Part model, mm, in its own coordinate system. Face numbers are marked on the shaded views. Coordinates: 2 decimals unless noted, no trailing zeros. Write each loop counter-clockwise with the first axis right and the second up, starting at its lowest first coordinate (ties: lowest second). Pieces come first, ordered by that corner, then holes. Notation, with made-up numbers: M 80.5,-28 L 132.5,-28 A35 cw 132.5,11 Z; hole C -34,58.25 d10. An arc over 180 degrees is marked long. Use a Markdown table: item, result. Add a question column.
Q1. Wall check: L1, parallel to Z at x = 20, y = -4.25; L2, parallel to Z at x = 18.5, y = -3; L3, parallel to Y at x = 96.5, z = -6. Give the ranges that are in metal, low to high. Write a range as from..to.
Q2. Slice it at A-A on x = 56.5. Write the cut outline in (y, z).
Q3. Mould opens along Z. For the marked faces 1, 2 and 3 say: released by +Z, released by -Z, zero draft, split by the parting line, or undercut.
Q4. Pin check, flat tips, straight feed: pin 1 Ø4 at (x, z) = (66, 4.5) entering from -Y; pin 2 Ø0.9 at (y, z) = (1, 5.5) entering from +X; pin 3 Ø3 at (x, y) = (61, -6) entering from +Z. Stop position of each tip, or through.
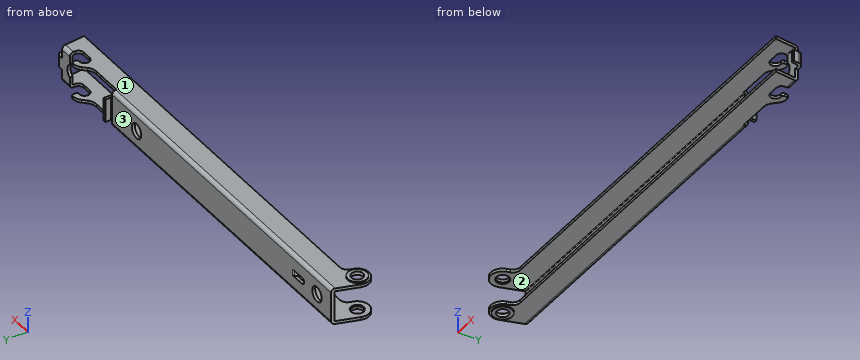
from build123d import *
from OCP.BRepFilletAPI import BRepFilletAPI_MakeFillet

# Parameters (mm, degrees)
BOSS_EXTRUDE1_DEPTH = 6.35
SKETCH2_R           = 3.2766
BOSS_EXTRUDE2_DEPTH = 0.381
FILLET1_R1          = 1.27
FILLET1_R2          = 2.54
SHELL1_T            = -1.016
BOSS_EXTRUDE3_DEPTH = 6.35
FILLET2_R           = 1.27
SHELL2_START        = 118.3386
SHELL2_DEPTH        = 27.813
SHELL2_START_2      = 129.293990182
SHELL2_2_DEPTH      = 7.764409818
FILLET3_R           = 0.635
SKETCH4_R           = 2.032
CUT_EXTRUDE1_DEPTH  = 148.431229717
EXTRUDE_THIN1_DEPTH = 2.0066
CUT_EXTRUDE2_DEPTH  = 150.225017324
EXTRUDE_THIN2_DEPTH = 4.0005
SKETCH8_R           = 2.54
CUT_EXTRUDE3_DEPTH  = 150.217877052
EXTRUDE_THIN3_DEPTH = 1.0795
FILLET4_R           = 0.635
FILLET6_RADIUS      = 1.0795
FILLET6_LENGTH      = 1.016


# Read off the part's stored shape, not the designer's step: Shell2
with BuildPart() as part:
    # Sketch1 → Boss-Extrude1 (new, symmetric)
    with BuildSketch(Plane.XY):
        with BuildLine():
            Line((0, 0), (118.3386, 0))
            Line((118.3386, 0), (118.3386, -8.128))
            Line((118.3386, -8.128), (5.974494608, -8.128))
            Line((5.974494608, -8.128), (5.047186378, -11.093494156))
            ThreePointArc((5.047186378, -11.093494156), (-0.044494156, -13.759386378), (-2.710386378, -8.667705844))
            Line((-2.710386378, -8.667705844), (0, 0))
        make_face()
    extrude(amount=BOSS_EXTRUDE1_DEPTH, both=True)

    # Sketch2 → Boss-Extrude2 (add)
    with BuildSketch(Plane.XY.offset(6.35)):
        with Locations(Location((1.1684, -9.8806, 0), (0, 0, 180))):
            Circle(SKETCH2_R)
    boss_extrude2 = extrude(amount=BOSS_EXTRUDE2_DEPTH)

    # Mirror1: Boss-Extrude2 across plane
    add(boss_extrude2.mirror(Plane.XY))

    # Fillet1: one fillet with a radius per group of edges: ONE call of the kernel's fillet builder (fillet() takes one radius for all edges)
    fillet1_edges_1 = [part.edges().sort_by_distance(p)[0] for p in [
        (59.1693, 0, 6.35),
        (59.1693, 0, -6.35),
    ]]
    fillet1_edges_2 = [part.edges().sort_by_distance(p)[0] for p in [
        (5.974494608, -8.128, 0),
    ]]
    fillet1 = BRepFilletAPI_MakeFillet(part.part.solid().wrapped)
    for e in fillet1_edges_1:
        fillet1.Add(FILLET1_R1, e.wrapped)
    for e in fillet1_edges_2:
        fillet1.Add(FILLET1_R2, e.wrapped)
    add(Compound.cast(fillet1.Shape()), mode=Mode.REPLACE)

    # Shell1
    shell1_openings = [part.faces().sort_by_distance(p)[0] for p in [
        (118.3386, -4.089523172, 0),
        (63.090062087, -8.128, 0),
        (5.232234532, -10.501717654, 0),
        (-0.044494156, -13.759386378, 0),
        (-1.363208192, -4.359484576, 0),
        (6.337175389, -8.621408996, 0),
    ]]
    offset(amount=SHELL1_T, openings=shell1_openings, kind=Kind.INTERSECTION)

    # Sketch3 → Boss-Extrude3 (add, symmetric)
    with BuildSketch(Plane.XY):
        with BuildLine():
            Line((118.3386, -8.128), (146.1516, -8.128))
            Line((146.1516, -8.128), (145.2626, 0.0762))
            Line((145.2626, 0.0762), (141.1224, 0.0762))
            Line((141.1224, 0.0762), (141.1224, -1.8034))
            ThreePointArc((141.1224, -1.8034), (140.594196369, -3.078596369), (139.319, -3.6068))
            Line((139.319, -3.6068), (136.0678, -3.6068))
            ThreePointArc((136.0678, -3.6068), (134.2644, -1.8034), (136.0678, 0))
            Line((136.0678, 0), (137.0584, 0))
            Line((137.0584, 0), (137.0584, 2.1082))
            Line((137.0584, 2.1082), (136.060885789, 2.1082))
            ThreePointArc((136.060885789, 2.1082), (134.588974152, 1.812396371), (133.345617268, 0.97091713))
            Line((133.345617268, 0.97091713), (132.009258703, -0.38671713))
            ThreePointArc((132.009258703, -0.38671713), (130.765901819, -1.228196371), (129.293990182, -1.524))
            Line((129.293990182, -1.524), (118.3386, -1.524))
            Line((118.3386, -1.524), (118.3386, -8.128))
        make_face()
    extrude(amount=BOSS_EXTRUDE3_DEPTH, both=True)

    # Fillet2
    fillet2_edges = [part.edges().sort_by_distance(p)[0] for p in [
        (143.1925, 0.0762, -6.35),
        (143.1925, 0.0762, 6.35),
    ]]
    fillet(fillet2_edges, radius=FILLET2_R)

    # Shell2 outline → Shell2 (cut)
    with BuildSketch(Plane.YZ.offset(SHELL2_START)):
        with BuildLine():
            Line((-8.128, 5.334), (-8.128, -5.334))
            Line((-8.128, -5.334), (-1.1938, -5.334))
            ThreePointArc((-1.1938, -5.334), (-1.014194878, -5.259605122), (-0.9398, -5.08))
            Line((-0.9398, -5.08), (-0.9398, 5.08))
            ThreePointArc((-0.9398, 5.08), (-1.014194878, 5.259605122), (-1.1938, 5.334))
            Line((-1.1938, 5.334), (-8.128, 5.334))
        make_face()
    extrude(amount=SHELL2_DEPTH, mode=Mode.SUBTRACT)

    # Shell2 2 outline → Shell2 2 (cut)
    with BuildSketch(Plane.YZ.offset(SHELL2_START_2)):
        with BuildLine():
            ThreePointArc((-1.1938, 5.334), (-1.014194878, 5.259605122), (-0.9398, 5.08))
            Line((-0.9398, 5.08), (-0.9398, -5.08))
            ThreePointArc((-0.9398, -5.08), (-1.014194878, -5.259605122), (-1.1938, -5.334))
            Line((-1.1938, -5.334), (2.1082, -5.334))
            Line((2.1082, -5.334), (2.1082, 5.334))
            Line((2.1082, 5.334), (-1.1938, 5.334))
        make_face()
    extrude(amount=SHELL2_2_DEPTH, mode=Mode.SUBTRACT)

    # Fillet3
    fillet3_edges = [part.edges().sort_by_distance(p)[0] for p in [
        (137.0584, 2.1082, -5.842),
        (137.0584, 0, -5.842),
        (137.0584, 0, 5.842),
        (137.0584, 2.1082, 5.842),
    ]]
    fillet(fillet3_edges, radius=FILLET3_R)

    # Sketch4 → Cut-Extrude1 (cut, through all)
    with BuildSketch(Plane.XY.offset(6.731)):
        with Locations((1.1684, -9.8806)):
            Circle(SKETCH4_R)
    extrude(amount=-CUT_EXTRUDE1_DEPTH, mode=Mode.SUBTRACT)

    # Sketch5 → Extrude-Thin1 (add, symmetric)
    with BuildSketch(Plane.XY):
        with BuildLine():
            Line((145.2626, 0.0762), (146.574836441, 0.0762))
            ThreePointArc((146.574836441, 0.0762), (147.677595365, -0.346091835), (148.216228196, -1.396940212))
            Line((148.216228196, -1.396940212), (148.412319576, -3.206583512))
            Line((148.412319576, -3.206583512), (147.402232341, -3.316035689))
            Line((147.402232341, -3.316035689), (147.206140962, -1.506392389))
            ThreePointArc((147.206140962, -1.506392389), (146.998974488, -1.102219937), (146.574836441, -0.9398))
            Line((146.574836441, -0.9398), (145.2626, -0.9398))
            Line((145.2626, -0.9398), (145.2626, 0.0762))
        make_face()
    extrude(amount=EXTRUDE_THIN1_DEPTH, both=True)

    # Sketch6 → Cut-Extrude2 (cut, through all)
    with BuildSketch(Plane(origin=(0, 0.0762, 0), x_dir=(1, 0, 0), z_dir=(0, 1, 0))):
        with BuildLine():
            Line((141.1224, 2.3495), (141.1224, -2.3495))
            ThreePointArc((141.1224, -2.3495), (142.3924, 0), (141.1224, 2.3495))
        make_face()
    extrude(amount=-CUT_EXTRUDE2_DEPTH, mode=Mode.SUBTRACT)

    # Sketch7 → Extrude-Thin2 (add, symmetric)
    with BuildSketch(Plane.XY):
        with BuildLine():
            ThreePointArc((118.3386, -1.016), (119.236625612, -0.644025612), (119.6086, 0.254))
            Line((119.6086, 0.254), (119.6086, 2.159))
            Line((119.6086, 2.159), (118.5926, 2.159))
            Line((118.5926, 2.159), (118.5926, 0.254))
            ThreePointArc((118.5926, 0.254), (118.518205122, 0.074394878), (118.3386, 0))
            Line((118.3386, 0), (118.3386, -1.016))
        make_face()
    extrude(amount=EXTRUDE_THIN2_DEPTH, both=True)

    # Sketch8 → Cut-Extrude3 (cut, through all)
    with BuildSketch(Plane(origin=(0, 0, 0), x_dir=(1, 0, 0), z_dir=(0, 1, 0))):
        with Locations(Location((7.556297414, 0, 0), (0, 0, 270))):
            Circle(SKETCH8_R)
        with Locations(Location((105.1306, 0, 0), (0, 0, 270))):
            Circle(SKETCH8_R)
        with BuildLine():
            Line((20.891297414, -1.0795), (20.891297414, 1.0795))
            Line((20.891297414, 1.0795), (15.620797414, 1.0795))
            ThreePointArc((15.620797414, 1.0795), (14.541297414, 0), (15.620797414, -1.0795))
            Line((15.620797414, -1.0795), (20.891297414, -1.0795))
        make_face()
    extrude(amount=-CUT_EXTRUDE3_DEPTH, mode=Mode.SUBTRACT)

    # Sketch9 → Extrude-Thin3 (add, symmetric)
    with BuildSketch(Plane.XY):
        Polygon((21.907297414, -1.016), (20.891297414, -1.016), (19.240297016, -3.3782), (14.795297016, -3.3782), (14.795297016, -2.3622), (18.710844734, -2.3622), (20.361845133, 0), (21.907297414, 0), align=None)
    extrude(amount=EXTRUDE_THIN3_DEPTH, both=True)

    # Fillet4
    fillet4_edges = [part.edges().sort_by_distance(p)[0] for p in [
        (20.891297414, -1.016, 0),
        (18.710844734, -2.3622, 0),
        (19.240297016, -3.3782, 0),
        (20.361845133, 0, 0),
    ]]
    fillet(fillet4_edges, radius=FILLET4_R)

    # Fillet6: full round fillet: the end face becomes a half cylinder, R = half its width
    fillet6_face = Plane((14.795297016, -2.8702, 0), x_dir=(0, -1, 0), z_dir=(-1, 0, 0))  # on the end face: x along it, z out of the body
    fillet6_slab = fillet6_face.offset(-FILLET6_RADIUS / 2) * Box(FILLET6_LENGTH, 2 * FILLET6_RADIUS, FILLET6_RADIUS, mode=Mode.PRIVATE)  # the body's end, R deep
    fillet6_round = Plane((15.874797016, -2.8702, 0), x_dir=(-1, 0, 0), z_dir=(0, -1, 0)) * Cylinder(FILLET6_RADIUS, FILLET6_LENGTH, mode=Mode.PRIVATE)  # its axis R under the face
    add(fillet6_slab - fillet6_round, mode=Mode.SUBTRACT)


solid = part.part
Recorded:
| question | item | result |
|---|---|---|
| 1 | L1 | -6.35..-5.33, 5.33..6.35 |
| 1 | L2 | -6.35..-5.33, -1.08..1.08, 5.33..6.35 |
| 1 | L3 | -8.13..-0.39 |
| 2 | outline | M -8.13,-6.35 L -1.27,-6.35 A1.27 ccw 0,-5.08 L 0,5.08 A1.27 ccw -1.27,6.35 L -8.13,6.35 L -8.13,5.33 L -1.27,5.33 A0.25 cw -1.02,5.08 L -1.02,-5.08 A0.25 cw -1.27,-5.33 L -8.13,-5.33 Z |
| 3 | face 1 | released by +Z |
| 3 | face 2 | undercut |
| 3 | face 3 | zero draft |
| 4 | pin 1 | y = -8.13 |
| 4 | pin 2 | x = 137.06 |
| 4 | pin 3 | z = 6.35 |
